Here's how the part is built. I have some questions about the finished solid (model axes, mm). Face numbers are marked on the shaded views. A direction names the side the tool comes from. Give positions to 0.01 mm unless a question says otherwise; leave off trailing zeros. Write each loop counter-clockwise with the first axis right and the second up, starting at its lowest first coordinate (ties: lowest second). Pieces come first, ordered by that corner, then holes. Notation, with made-up numbers: (44.5, 71) - (98.5, 71) arc R25 cw to (98.5, 88) - close; hole circle Ø11 at (-15, 29). An arc over 180 degrees is marked (long way). Use one line per item in the form item = value. Start each with the question number.
from build123d import *

# Parameters (mm, degrees)
F0_R     = 13.4462075072
F1_DEPTH = 50.8
F0_R_2   = 15.1279388752
F2_DEPTH = 51.816
F0_R_3   = 17.8416483947
F3_DEPTH = 28.956
F4_START = 17.526
F4_DEPTH = 7.62


with BuildPart() as f1:
    # F0 (on Top) → F1 (new body)
    with BuildSketch(Plane.XY):
        Circle(F0_R)
    extrude(amount=F1_DEPTH)

    # F0 (on Top) → F2 (join)
    with BuildSketch(Plane.XY):
        Circle(F0_R_2)
        Circle(F0_R, mode=Mode.SUBTRACT)
    extrude(amount=F2_DEPTH)

    # F0 (on Top) → F3 (join)
    with BuildSketch(Plane.XY):
        Circle(F0_R_3)
        Circle(F0_R_2, mode=Mode.SUBTRACT)
    extrude(amount=F3_DEPTH)

    # F0 (on Top) → F4 (join)
    with BuildSketch(Plane.XY.offset(F4_START)):
        Polygon((21.8152726681, 5.6546813213), (11.4272637293, 19.4241907448), (-5.6546813213, 21.8152726681), (-19.4241907448, 11.4272637293), (-21.8152726681, -5.6546813213), (-11.4272637293, -19.4241907448), (5.6546813213, -21.8152726681), (19.4241907448, -11.4272637293), align=None)
        Circle(F0_R_3, mode=Mode.SUBTRACT)
    extrude(amount=F4_DEPTH)


solid = f1.part
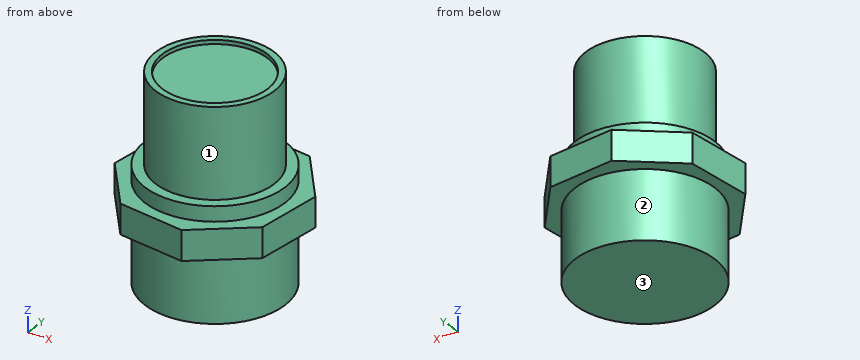
1. For the marked faces 1, 2 and 3, which set-ups out of +Z, -Z, +X, -X, +Y, -Y let a thin tool reach every point of the face, with its end or its side?
2. I want a section at A-A, the plane z = 3.5. List the corners of the cut face in (x, y) for me.
3. I want a section at B-B, the plane x = 16.5. List the corners of the cut face in (y, z) for me.
4. I want a section at C-C, the plane y = 0. List the corners of the cut face in (x, z) for me, then the cut area to 3 significant figures.
5. I want a section at D-D, the plane z = 41.5. List the corners of the cut face in (x, y) for me.
6. Please list where these lines run through material, in increasing order: line 1 (Y direction, x = 0, z = 51.4); line 2 (Z direction, x = -5, y = -16); line 3 (Z direction, x = 6.5, y = 19.5).
7. For P1, Ø6, axis at x = 6.5, z = 34, coming from the -Y side; P2, Ø8, axis at y = 12.5, z = 23.5, coming from the -X side; P3, Ø8, axis at x = 4.5, z = 31.5, coming from the -Y side, each with a flat end and sliding along its axis, tell me the tip position at first contact or that it passes through.
Result sheet:
q1.face_1 = +Z
q1.face_2 = -Z
q1.face_3 = -Z, +X, -X, +Y, -Y
q2.outline = circle Ø35.68 at (0, 0)
q3.outline = (-13.63, 17.53) - (-6.79, 17.53) - (-6.79, 0) - (6.79, 0) - (6.79, 17.53) - (12.7, 17.53) - (12.7, 25.15) - (6.79, 25.15) - (6.79, 28.96) - (-6.79, 28.96) - (-6.79, 25.15) - (-13.63, 25.15) - close
q4.outline = (-21.02, 17.53) - (-17.84, 17.53) - (-17.84, 0) - (17.84, 0) - (17.84, 17.53) - (21.02, 17.53) - (21.02, 25.15) - (17.84, 25.15) - (17.84, 28.96) - (15.13, 28.96) - (15.13, 51.82) - (13.45, 51.82) - (13.45, 50.8) - (-13.45, 50.8) - (-13.45, 51.82) - (-15.13, 51.82) - (-15.13, 28.96) - (-17.84, 28.96) - (-17.84, 25.15) - (-21.02, 25.15) - close
q4.area = 1,750 mm2
q5.outline = circle Ø30.26 at (0, 0)
q6.line_1 = -15.13 to -13.45, 13.45 to 15.13
q6.line_2 = 0 to 28.96
q6.line_3 = 17.53 to 25.15
q7.P1 = -14.72
q7.P2 = -19.83
q7.P3 = -17.79
